Verification items for this drawing (mm, ordinates from the low corner). Round coordinates to 2 decimals unless told otherwise and drop trailing zeros. Loops run counter-clockwise (first coordinate to the right, second up) from the corner with the lowest first, then second, coordinate; pieces in that order, holes last. Notation, with made-up numbers: (63.25, -32.75) - (104.25, -32.75) arc R18 ccw to (104.25, -5.75) - close; hole circle Ø2 at (22.25, 82). An arc over 180 degrees is marked (long way). Answer in a Markdown table with one row per item. Add a question column.
(1) Gauge pin test, flat end, axial feed: pin 1 (2.5 mm diameter, centred on x = 14, z = 15, fed in from +Y). Record the tip position at first contact, or that the pin passes through.
(2) Cross-section at A-A on x = 14. Enter the section's corners in (y, z) (3 decimals).
(3) Mould release check, pull along X, two halves, no side actions. Record for the marked faces 1, 2 and 3: +X half, -X half, draft (parallel to the pull), parting line (faces both ways), or undercut.
(4) Cross-section at B-B on y = 0.5. Enter the section's corners in (x, z) (3 decimals), then the cut area to 3 significant figures.
(5) Thickness scan on line 1 along Z through (x, y) = (14, 5.5) (3 decimals); line 2 along X through (y, z) = (9.85, 14) (3 decimals). Record the ranges inside material, lowest first.
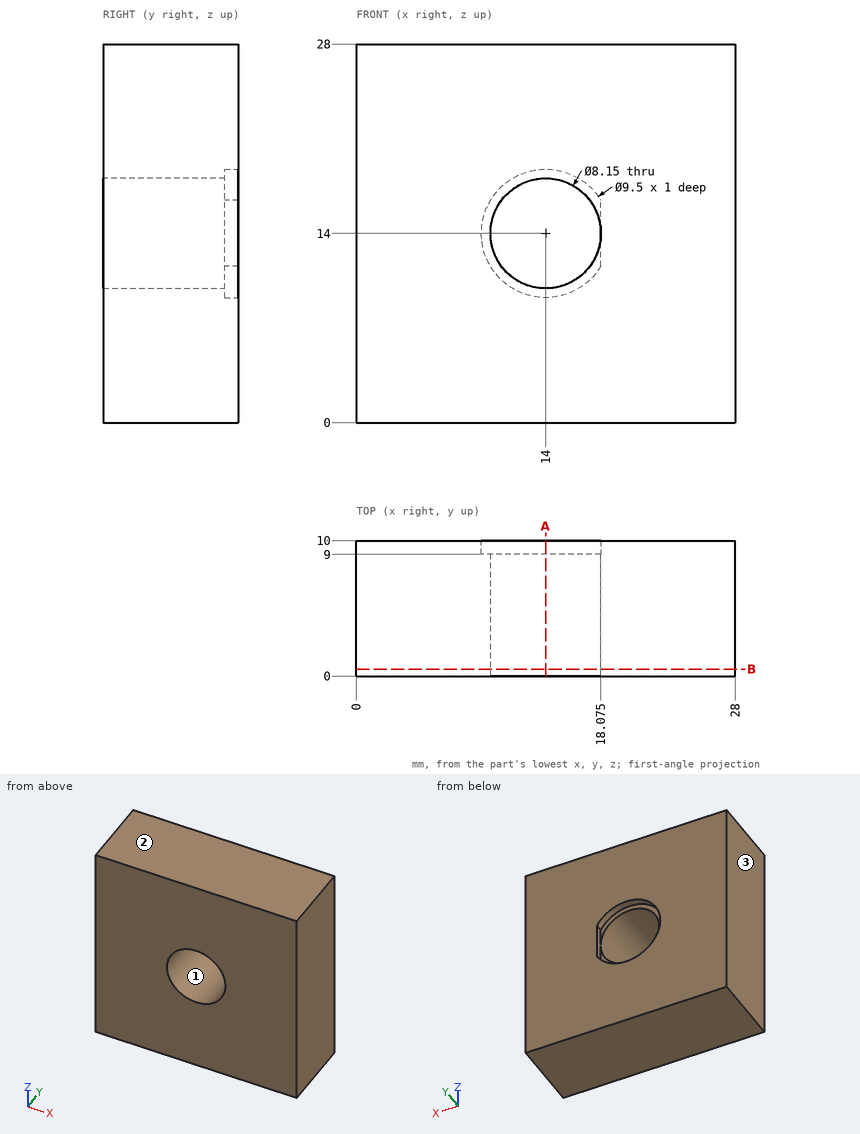
Answers:
| question | item | result |
|---|---|---|
| 1 | pin 1 | passes through |
| 2 | outline | (0, 0) - (10, 0) - (10, 9.25) - (9, 9.25) - (9, 9.925) - (0, 9.925) - close; (0, 18.075) - (9, 18.075) - (9, 18.75) - (10, 18.75) - (10, 28) - (0, 28) - close |
| 3 | face 1 | undercut |
| 3 | face 2 | draft |
| 3 | face 3 | -X half |
| 4 | outline | (0, 0) - (28, 0) - (28, 28) - (0, 28) - close; hole circle Ø8.15 at (14, 14) |
| 4 | area | 732 mm^2 |
| 5 | line 1 | z = 0 to 9.925, 18.075 to 28 |
| 5 | line 2 | x = 0 to 9.25, 18.075 to 28 |
